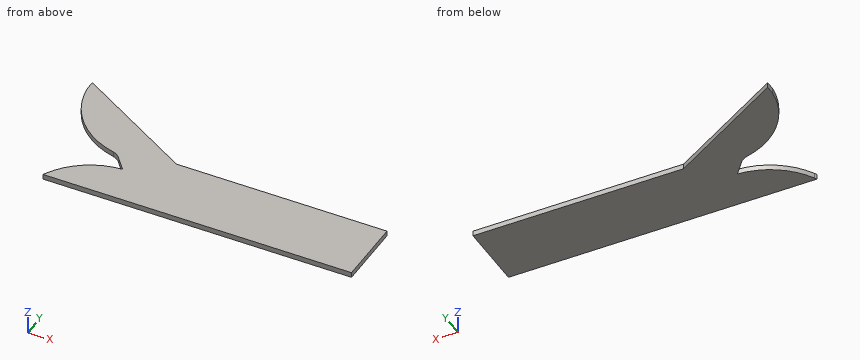
```python
from build123d import *

# Parameters (mm, degrees)
BOSS_EXTRUDE1_DEPTH = 33.45
CAVITY3_DEPTH       = 33.45
CUT_EXTRUDE2_REACH  = 1606.713


# Read off the part's stored shape, not the designer's step: Cavity3
with BuildPart() as part:
    # Sketch1 → Boss-Extrude1 (new body)
    with BuildSketch(Plane.XY):
        Polygon((-678.5, 219.25), (-1456.5, 672.75), (-1456.5, -219.25), (-678.5, -219.25), (678.5, -219.25), (678.5, 219.25), align=None)
    extrude(amount=BOSS_EXTRUDE1_DEPTH)

    # Cavity3 outline → Cavity3 (cut)
    with BuildSketch(Plane.XY):
        with BuildLine():
            Line((-1456.5, -202.506493086), (-1300.878272365, -202.506493086))
            ThreePointArc((-1300.878272365, -202.506493086), (-1145.343683701, -35.513747144), (-927.890567992, 33.708560944))
            Line((-927.890567992, 33.708560944), (-994.109648548, 112.218170508))
            ThreePointArc((-994.109648548, 112.218170508), (-1017.687293376, 137.407064936), (-1048.421985466, 153.083940911))
            ThreePointArc((-1048.421985466, 153.083940911), (-1325.171989397, 317.426039094), (-1456.5, 611.282881012))
            Line((-1456.5, 611.282881012), (-1456.5, -202.506493086))
        make_face()
    extrude(amount=CAVITY3_DEPTH, mode=Mode.SUBTRACT)

    # Sketch6 → Cut-Extrude2 (cut, up to next)
    with BuildSketch(Plane.XY.offset(33.45), mode=Mode.PRIVATE) as cut_extrude2_sk1:
        with BuildLine():
            Line((-1300.878272365, -202.506493086), (-1456.5, -202.506493086))
            Line((-1456.5, -202.506493086), (-1456.5, -219.25))
            Line((-1456.5, -219.25), (-1309.43889328, -219.25))
            ThreePointArc((-1309.43889328, -219.25), (-1305.246054091, -210.833524229), (-1300.878272365, -202.506493086))
        make_face()
    cut_extrude2_tool1 = extrude(cut_extrude2_sk1.sketch, amount=-CUT_EXTRUDE2_REACH, mode=Mode.PRIVATE) & part.part
    add(cut_extrude2_tool1.solids().sort_by_distance((-1380.845886, -210.799292, 33.45))[0], mode=Mode.SUBTRACT)


solid = part.part
```
Geometry: final body of the model. Coordinates: model frame, mm. Round coordinates to 2 decimals unless told otherwise and drop trailing zeros. Write each loop counter-clockwise with the first axis right and the second up, starting at its lowest first coordinate (ties: lowest second). Pieces come first, ordered by that corner, then holes. Notation, with made-up numbers: (-11, -10.5) -> (36, -10.5) arc R14 ccw to (36, 16.5) -> close; hole circle Ø10 at (85.25, -23). An arc over 180 degrees is marked (long way). Use CSV: the item, a comma, the result in double quotes. Start each with the question number.
Q1. Section B-B (z = 5.5). Return loops of the section in (x, y), plus the area to 3 significant figures.
Q2. First-contact query: pin 1 Ø6 at (x, z) = (-290, 8.5) entering from +Y; pin 2 Ø2 at (y, z) = (464.5, 25.5) entering from -X; pin 3 Ø4 at (x, y) = (-1192, -118) entering from -Z; pin 4 Ø12 at (y, z) = (45.5, 12) entering from -X. Flat tips, straight axial feed; report the tip coordinate or a pass-through.
Q3. Line query: L1, parallel to Y at x = 341, z = 9; L2, parallel to Y at x = -1002, z = 18; L3, parallel to X at y = 298.5, z = 22.5. Output: solid intervals per line, ascending.
Q4. Section A-A (x = -1151). Return loops of the section in (y, z), plus the area to 3 significant figures.
Q5. Section D-D (y = -5). Return loops of the section in (x, z).
Q6. Section C-C (x = 37.5). Return loops of the section in (y, z).
Result sheet:
1,outline,"(-1456.5, 611.28) arc R532 ccw to (-1048.42, 153.08) arc R100 cw to (-994.11, 112.22) -> (-927.89, 33.71) arc R450 ccw to (-1300.88, -202.51) arc R450 ccw to (-1309.44, -219.25) -> (678.5, -219.25) -> (678.5, 219.25) -> (-678.5, 219.25) -> (-1456.5, 672.75) -> close"
1,area,"937,000 mm²"
2,pin 1,"y = 219.25"
2,pin 2,"x = -1418.49"
2,pin 3,"z = 0"
2,pin 4,"x = -942.9"
3,L1,"-219.25 to 219.25"
3,L2,"-219.25 to 23.64, 122.71 to 407.82"
3,L3,"-1307.47 to -814.46"
4,outline,"(-219.25, 0) -> (-39.16, 0) -> (-39.16, 33.45) -> (-219.25, 33.45) -> close; (188.29, 0) -> (494.67, 0) -> (494.67, 33.45) -> (188.29, 33.45) -> close"
4,area,"16,300 mm²"
5,outline,"(-1088.52, 0) -> (678.5, 0) -> (678.5, 33.45) -> (-1088.52, 33.45) -> close"
6,outline,"(-219.25, 0) -> (219.25, 0) -> (219.25, 33.45) -> (-219.25, 33.45) -> close"
